Verification items for this drawing (mm, ordinates from the low corner). A direction names the side the tool comes from. Round coordinates to 2 decimals unless told otherwise and drop trailing zeros. Write each loop counter-clockwise with the first axis right and the second up, starting at its lowest first coordinate (ties: lowest second). Pieces come first, ordered by that corner, then holes.
Item 1: Depth check by flat-ended pin: P1, Ø4, axis at x = 9.525, z = 6.35, coming from the -Y side. Enter the tip coordinate at first touch or a pass-through.
Item 2: Cross-section at C-C (y = 11.5). Enter the section's corners in (x, z) (3 decimals), then the cut area to 3 significant figures.
Item 3: Access from +Z, -Z, +X, -X, +Y, -Y to the whole of each face (thin tool, end or side, straight path). Record for the marked faces 4 and 5.
Item 4: Scan lines: probe 1 along X at (y, z) = (2.2, 6.35) (3 decimals); probe 2 along Y at (x, z) = (2.2, 6.35) (3 decimals); probe 3 along X at (y, z) = (14, 9) (3 decimals). Record each from-to range of solid material in increasing order.
Item 5: Cross-section at B-B (x = 20). Enter the section's corners in (y, z) (3 decimals), then the cut area to 3 significant figures.
Item 6: Draft check along Z on the marked faces 1, 2 and 3. Enter one of: pulls with the +Z half, pulls with the -Z half, needs draft (parallel to the pull), parting line crosses it, or undercut.
Item 7: Cross-section at D-D (y = 15). Enter the section's corners in (x, z) (3 decimals), then the cut area to 3 significant figures.
Item 8: Cross-section at A-A (z = 6.35). Enter the section's corners in (x, y) (3 decimals), then the cut area to 3 significant figures.
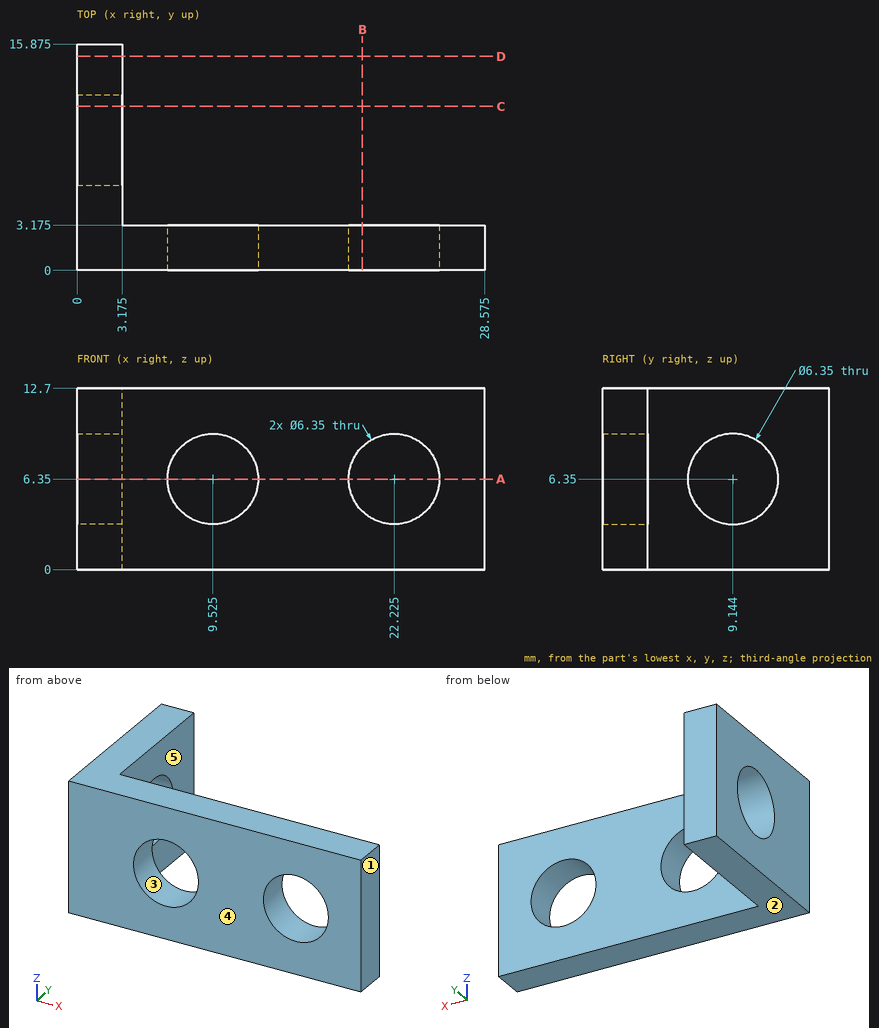
Resolved:
1. P1: passes through
2. outline: (0, 0) - (3.175, 0) - (3.175, 4.222) - (0, 4.222) - close; (0, 8.478) - (3.175, 8.478) - (3.175, 12.7) - (0, 12.7) - close
2. area: 26.8 mm2
3. face 4: +Z, -Z, +X, -X, -Y
3. face 5: +Z, -Z, +X, +Y
4. probe 1: x = 0 to 6.35, 12.7 to 19.05, 25.4 to 28.575
4. probe 2: y = 0 to 5.969, 12.319 to 15.875
4. probe 3: x = 0 to 3.175
5. outline: (0, 0) - (3.175, 0) - (3.175, 4.085) - (0, 4.085) - close; (0, 8.615) - (3.175, 8.615) - (3.175, 12.7) - (0, 12.7) - close
5. area: 25.9 mm2
6. face 1: needs draft
6. face 2: pulls with the -Z half
6. face 3: undercut
7. outline: (0, 0) - (3.175, 0) - (3.175, 12.7) - (0, 12.7) - close
7. area: 40.3 mm2
8. outline: (0, 0) - (6.35, 0) - (6.35, 3.175) - (3.175, 3.175) - (3.175, 5.969) - (0, 5.969) - close; (0, 12.319) - (3.175, 12.319) - (3.175, 15.875) - (0, 15.875) - close; (12.7, 0) - (19.05, 0) - (19.05, 3.175) - (12.7, 3.175) - close; (25.4, 0) - (28.575, 0) - (28.575, 3.175) - (25.4, 3.175) - close
8. area: 70.6 mm2
